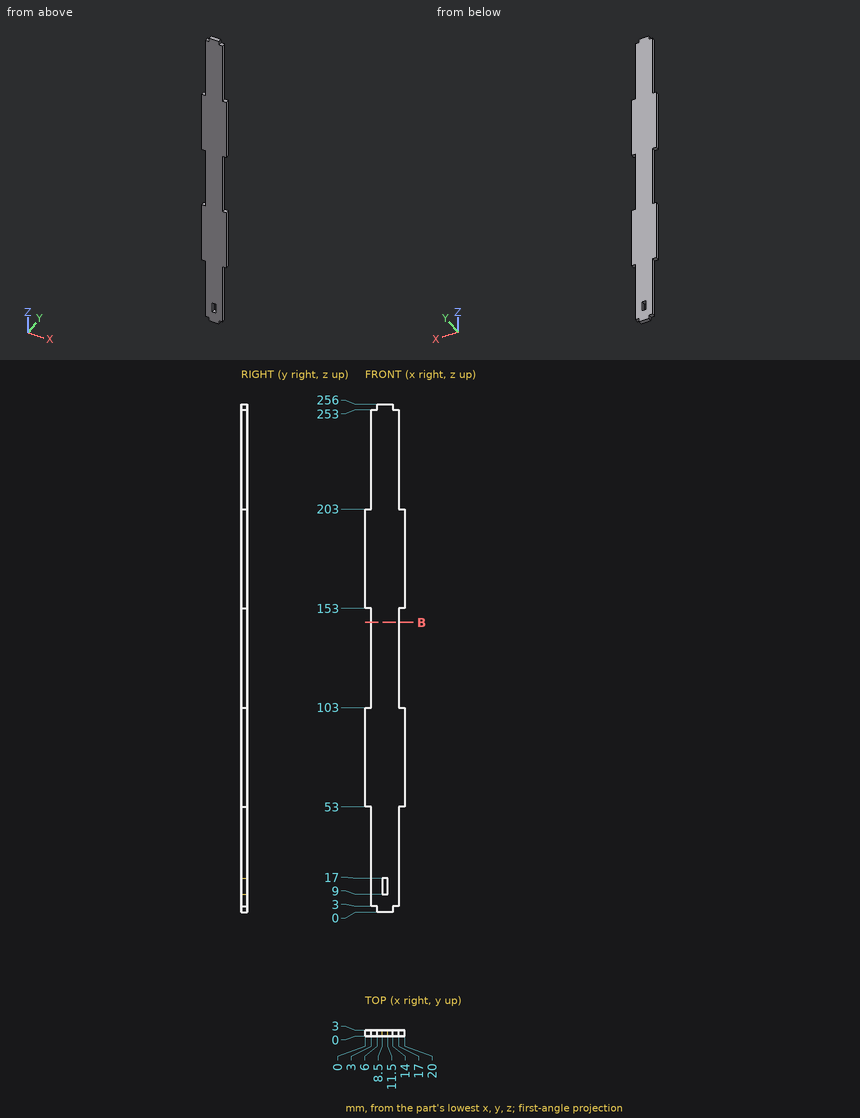
Study the drawing (mm; zero at the part's minimum x, y, z) and answer. Coordinates: 2 decimals unless noted, no trailing zeros. Write each loop counter-clockwise with the first axis right and the second up, starting at its lowest first coordinate (ties: lowest second). Pieces come first, ordered by that corner, then holes. Notation, with made-up numbers: M 2.25,83 L 6.25,83 A15 cw 6.25,90 Z; hole C 54,-32.75 d7. An arc over 180 degrees is marked long. Use a Markdown table: item, result. Add a question column.
1. Straight lines are drawn through the part: line 1 along Z through (x, y) = (10.25, 2.55); line 2 along X through (y, z) = (0.5, 12.5); line 3 along Z through (x, y) = (17.75, 1.65). For each, find the intervals that lie inside material, in ascending order. Write a range as [from, to].
2. Given P1, Ø0.9, axis at y = 1, z = 20, coming from the +X side; P2, Ø1.5, axis at x = 18, y = 1.5, coming from the -Z side; P3, Ø1, axis at x = 8.5, z = 50, coming from the -Y side; P4, Ø1.5, axis at x = 15, y = 1.5, coming from the +Z side, each flat-ended and moving along its own axis, determine where each tip first touches the part or whether it passes through.
3. Section B-B (z = 146) is taken. Give the vertices of the cut face in (x, y), plus the area to 3 significant figures.
Data:
| question | item | result |
|---|---|---|
| 1 | line 1 | z = [0, 9], [17, 256] |
| 1 | line 2 | x = [3, 8.5], [11.5, 17] |
| 1 | line 3 | z = [53, 103], [153, 203] |
| 2 | P1 | stops at x = 17 |
| 2 | P2 | stops at z = 53 |
| 2 | P3 | stops at y = 0 |
| 2 | P4 | stops at z = 253 |
| 3 | outline | M 3,0 L 17,0 L 17,3 L 3,3 Z |
| 3 | area | 42.0 mm2 |
